Here's how the part is built. I have some questions about the finished solid (model axes, mm). A direction names the side the tool comes from. Coordinates: 2 decimals unless noted, no trailing zeros. Loops run counter-clockwise (first coordinate to the right, second up) from the corner with the lowest first, then second, coordinate; pieces in that order, holes last. Notation, with made-up numbers: (24, -5) -> (82, -5) arc R21 ccw to (82, 26) -> close; hole circle Ø6 at (72, 24). An arc over 180 degrees is marked (long way). Answer as a JSON object with one key per item and string values. Group by question number.
1) I need wall thicknesses on probe 1 along Z at (x, y) = (0, -2.95); probe 2 along Z at (x, y) = (0, -1.6); probe 3 along Y at (x, z) = (-7.5, 36). Which ranges of each line are inside material? Lowest first, please. Write a range as [from, to].
2) I want a section at B-B (x = 12). Write out the boundary of the cut face in (y, z), then the cut area to 3 significant figures.
3) I want a section at A-A (z = 39). Write out the boundary of the cut face in (x, y), then the cut area to 3 significant figures.
4) Which directions (+Z, -Z, +X, -X, +Y, -Y) give clear straight access to the entire face, cutting with the end or side of a thin tool? Please do faces 1 (the cylindrical face through (3.15, -6.86, 23.85)), 2 (the cylindrical face through (-17.357, -2.439, 43.138)).
5) If we mould it in two halves opening along Z, with no side actions, what happens to faces 3 (the cylindrical face through (-17.357, -5.903, 45.966)), 4 (the flat face through (-17.5, -4, 24)), 5 (the flat face through (0, -5, 18.5))? For each: +Z half, -Z half, draft (parallel to the pull), parting line (faces both ways), or undercut.
6) I want a section at C-C (x = 0). Count the separate pieces of the cut face and the enclosed holes in it, then the cut area to 3 significant figures.
7) I'm going to push flat-ended pins straight in: pin 1 (2 mm diameter, centred on x = 1.5, z = 4.5, fed in from -Y); pin 2 (17 mm diameter, centred on x = 4.5, z = 10.5, fed in from -Y); pin 3 (3 mm diameter, centred on x = 1, y = -5.5, fed in from +Z). Where does each tip first touch, or does it pass through?
```python
from build123d import *

# Parameters (mm, degrees)
F0_W     = 35
F0_H     = 41
F0_R     = 1.7
F1_DEPTH = 7
F3_DEPTH = 35
F4_R     = 1.7
F5_DEPTH = 3
F6_R     = 0.5


with BuildPart() as f1:
    # F0 (on Front) → F1 (new body)
    with BuildSketch(Plane.XZ):
        with Locations((0, 20.5)):
            Rectangle(F0_W, F0_H)
        with Locations((0, 6)):
            Circle(F0_R, mode=Mode.SUBTRACT)
        with Locations((0, 22)):
            Circle(F0_R, mode=Mode.SUBTRACT)
    extrude(amount=F1_DEPTH)

    # F2 (on face) → F3 (join, through all)
    with BuildSketch(Plane.YZ.offset(17.5)):
        Polygon((-10, 42.732051), (-7, 41), (0, 41), (-4.5, 45.330127), (-7.5, 47.062178), align=None)
    extrude(amount=-F3_DEPTH)

    # F4 (on face) → F5 (cut)
    with BuildSketch(Plane.XZ.offset(7)):
        Polygon((4.041452, 22), (2.020726, 25.5), (-2.020726, 25.5), (-4.041452, 22), (-2.020726, 18.5), (2.020726, 18.5), align=None)
        with Locations((0, 22)):
            Circle(F4_R, mode=Mode.SUBTRACT)
        Polygon((4.041452, 6), (2.020726, 9.5), (-2.020726, 9.5), (-4.041452, 6), (-2.020726, 2.5), (2.020726, 2.5), align=None)
        with Locations((0, 6)):
            Circle(F4_R, mode=Mode.SUBTRACT)
    extrude(amount=-F5_DEPTH, mode=Mode.SUBTRACT)

    # F6
    f6_edges = [f1.edges().sort_by_distance(p)[0] for p in [
        (17.5, -3.5, 0),
        (17.5, -7, 20.5),
        (17.5, -8.5, 41.866025),
        (17.5, -8.75, 44.897114),
        (17.5, -6, 46.196152),
        (17.5, -2.25, 43.165064),
        (17.5, 0, 20.5),
        (-17.5, -7, 20.5),
        (0, -7, 41),
        (0, -7, 0),
        (3.031089, -7, 7.75),
        (0, -7, 9.5),
        (-3.031089, -7, 7.75),
        (-3.031089, -7, 4.25),
        (0, -7, 2.5),
        (3.031089, -7, 4.25),
        (3.031089, -7, 20.25),
        (3.031089, -7, 23.75),
        (0, -7, 25.5),
        (-3.031089, -7, 23.75),
        (-3.031089, -7, 20.25),
        (0, -7, 18.5),
        (0, -7.5, 47.062178),
        (0, -10, 42.732051),
        (-17.5, -8.75, 44.897114),
        (-17.5, -3.5, 0),
        (-17.5, 0, 20.5),
        (-17.5, -2.25, 43.165064),
        (-17.5, -6, 46.196152),
        (-17.5, -8.5, 41.866025),
        (0, 0, 0),
        (0, 0, 41),
        (-1.7, 0, 6),
        (-1.7, 0, 22),
        (0, -4.5, 45.330127),
    ]]
    fillet(f6_edges, radius=F6_R)


solid = f1.part
```
Determined:
{
 "1": {"probe 1": "[0, 4.3], [7.7, 20.3], [23.7, 43.84]", "probe 2": "[0, 4.3], [7.7, 20.3], [23.7, 42.54]", "probe 3": "[-7, 0]"},
 "2": {"outline": "(-9.75, 43.17) arc R0.5 ccw to (-9.57, 42.48) -> (-7.25, 41.14) arc R0.5 cw to (-7, 40.71) -> (-7, 0.5) arc R0.5 ccw to (-6.5, 0) -> (-0.5, 0) arc R0.5 ccw to (0, 0.5) -> (0, 40.79) arc R0.5 ccw to (-0.15, 41.15) -> (-4.46, 45.29) arc R0.5 ccw to (-4.55, 45.36) -> (-7.07, 46.81) arc R0.5 ccw to (-7.75, 46.63) -> close", "area": "319 mm^2"},
 "3": {"outline": "(-17.5, -6.5) arc R0.5 ccw to (-17, -7) -> (17, -7) arc R0.5 ccw to (17.5, -6.5) -> (17.5, -0.5) arc R0.5 ccw to (17, 0) -> (-17, 0) arc R0.5 ccw to (-17.5, -0.5) -> close", "area": "245 mm^2"},
 "4": {"face 1": "-Y", "face 2": "+Z, -X, +Y"},
 "5": {"face 3": "+Z half", "face 4": "draft", "face 5": "undercut"},
 "6": {"separate pieces": "3", "enclosed holes": "0", "area": "250 mm^2"},
 "7": {"pin 1": "y = -4", "pin 2": "y = -7", "pin 3": "z = 46.77"}
}
